Autodesk Inventor part; units mm, degrees
ref_plane "YZ Plane" through (0, 0, 0) normal (1, 0, 0) x (0, 1, 0)
ref_plane "XZ Plane" through (0, 0, 0) normal (0, 1, 0) x (-1, 0, 0)
ref_plane "XY Plane" through (0, 0, 0) normal (0, 0, 1) x (1, 0, 0)
sketch "Sketch1" plane through (0, 0, 0) normal (0, 1, 0) x (-1, 0, 0)
  point P0 (0, 0)
sketch "Sketch2" plane through (0, 0, 0) normal (0, 1, 0) x (-1, 0, 0)
  line L0 (0, 0) -> (-30, 0)
  line L1 (-30, 0) -> (-30, -30)
  line L2 (-30, -30) -> (0, -30)
  line L3 (0, -30) -> (0, 0)
  line L4 (0, -30) -> (-30, 0) construction
  line L5 (0, 0) -> (-30, -30) construction
  line L6 (-15, -15) -> (0, -15) construction
  line L7 (-15, -15) -> (-30, -15) construction
  line L8 (-15, -15) -> (-15, -30) construction
  line L9 (-15, -15) -> (-15, 0) construction
  line L10 (-15, -15) -> (-9.25, -15) construction
  line L11 (-15, -17.4158) -> (-15, -15) construction
  line L12 (-15, -15) -> (-15, -20.75) construction
  line L13 (-15, -15) -> (-15, -9.25) construction
  line L14 (-15, -15) -> (-9.25, -15) construction
  line L15 (-15, -15) -> (-20.75, -15) construction
  line L16 (-15, -20.75) -> (-9.25, -15) construction
  line L17 (-9.25, -15) -> (-9.25, -20.75) construction
  line L18 (-9.25, -20.75) -> (-15, -20.75) construction
  line L19 (-15, -20.75) -> (-20.75, -20.75) construction
  line L20 (-20.75, -20.75) -> (-20.75, -15) construction
  line L21 (-9.25, -15) -> (-9.25, -9.25) construction
  line L22 (-15, -9.25) -> (-9.25, -9.25) construction
  line L23 (-15, -9.25) -> (-20.75, -9.25) construction
  line L24 (-20.75, -9.25) -> (-20.75, -15) construction
  line L25 (-15, -9.25) -> (-11, -9.25) construction
  line L26 (-15, -9.25) -> (-19, -9.25) construction
  line L27 (-11, -9.25) -> (-19, -9.25)
  line L28 (-11, -9.25) -> (-11, -3.25)
  line L29 (-11, -3.25) -> (-19, -3.25)
  line L30 (-19, -3.25) -> (-19, -9.25)
  line L31 (-11, -20.75) -> (-19, -20.75)
  line L32 (-19, -20.75) -> (-19, -26.75)
  line L33 (-19, -26.75) -> (-11, -26.75)
  line L34 (-11, -26.75) -> (-11, -20.75)
  line L35 (-9.25, -9.25) -> (-9.25, -10.75)
  line L36 (-9.25, -20.75) -> (-9.25, -18.75)
  line L37 (-9.25, -18.75) -> (-9.25, -19.25)
  line L38 (-9.25, -18.75) -> (-9.25, -10.75)
  line L39 (-9.25, -10.75) -> (-3.25, -10.75)
  line L40 (-3.25, -10.75) -> (-3.25, -18.75)
  line L41 (-3.25, -18.75) -> (-9.25, -18.75)
  line L42 (-9.25, -19.25) -> (-20.75, -19.25) construction
  line L43 (-20.75, -19.25) -> (-20.75, -11.25)
  line L44 (-20.75, -11.25) -> (-26.75, -11.25)
  line L45 (-26.75, -11.25) -> (-26.75, -19.25)
  line L46 (-26.75, -19.25) -> (-20.75, -19.25)
  line L47 (-9.25, -18.75) -> (-11.75, -18.75) construction
  line L48 (-11.75, -18.75) -> (-11.75, -10.75) construction
  line L49 (-11.75, -10.75) -> (-9.25, -10.75) construction
  line L50 (-20.75, -19.25) -> (-18.25, -19.25) construction
  line L51 (-18.25, -19.25) -> (-18.25, -11.25) construction
  line L52 (-18.25, -11.25) -> (-20.75, -11.25) construction
  line L53 (-9.25, -10.75) -> (-9.25, -11.75) construction
  line L54 (-9.25, -11.75) -> (-11.75, -11.75) construction
  line L55 (-20.75, -11.25) -> (-20.75, -11.75) construction
  line L56 (-20.75, -11.75) -> (-18.25, -11.75) construction
  line L57 (-11.75, -18.75) -> (-20.75, -18.75) construction
  line L58 (-18.25, -18.75) -> (-18.25, -11.75) construction
  line L59 (-15, -18.75) -> (-14.25, -18.75) construction
  line L60 (-15, -18.75) -> (-15.75, -18.75) construction
  line L61 (-11.75, -18.75) -> (-11.75, -11.75)
  line L62 (-11.75, -18.75) -> (-14.25, -18.75)
  line L63 (-11.75, -11.75) -> (-14.25, -11.75)
  line L64 (-15.75, -18.75) -> (-18.25, -18.75)
  line L65 (-18.25, -18.75) -> (-18.25, -11.75)
  line L66 (-18.25, -11.75) -> (-15.75, -11.75)
  line L67 (-14.25, -11.75) -> (-15.75, -11.75)
  line L68 (-14.25, -18.75) -> (-15.75, -18.75)
  dimension "d0" = 30
  dimension "d1" = 30
  dimension "d3" = 5.75
  dimension "d4" = 5.75
  dimension "d5" = 5.75
  dimension "d6" = 5.75
  dimension "d7" = 4
  dimension "d8" = 4
  dimension "d9" = 6
  dimension "d10" = 6
  dimension "d11" = 8
  dimension "d12" = 1.5
  dimension "d13" = 2
  dimension "d14" = 0.5
  dimension "d15" = 6
  dimension "d16" = 8
  dimension "d17" = 6
  dimension "d18" = 2.5
  dimension "d19" = 2.5
  dimension "d20" = 1
  dimension "d21" = 0.75
  dimension "d22" = 0.75
extrude "Extrusion1" add sketch "Sketch2" against normal blind 5 contours L3 L2 L1 L0 | L62 L68 L64 L65 L66 L67 L63 L61
extrude "Extrusion5" cut sketch "Sketch2" against normal blind 4 contours L62 L68 L64 L65 L66 L67 L63 L61
properties part number "switch_test_v1_3DPrint"
Read the model definition and answer for the solid it produces. Units are mm, in the model's axes. A direction names the side the tool comes from. Give positions to 0.01 mm unless a question says otherwise; leave off trailing zeros. Write each loop counter-clockwise with the first axis right and the second up, starting at its lowest first coordinate (ties: lowest second). Pieces come first, ordered by that corner, then holes. Notation, with made-up numbers: (-38.75, 9.25) - (-33.75, 9.25) arc R10 ccw to (-33.75, 13.25) - close; hole circle Ø4 at (33.5, -12.75). An arc over 180 degrees is marked (long way). Answer in a Markdown table with one row per item. Add a question column.
Item 1: Determine the mould class of faces 1 (the face through (15, -2, 0)), 2 (the face through (30, -2, -15)), 3 (the face through (6, -2, -10.75)) for opening direction X: pulls with the +X half, pulls with the -X half, needs draft (parallel to the pull), parting line crosses it, or undercut.
Item 2: A tool of negligible diameter and unlimited length cuts with its end or side. For faces 4 (the face through (11, -2, -24)), 5 (the face through (15, -5, -15)), 6 (the face through (15, -2, -11.75)), from which of +Z, -Z, +X, -X, +Y, -Y can it reach the whole face along a straight path? Write none if from no direction.
Item 3: Section C-C, the plane x = 24.25 is taken. Write down the section's boundary in (y, z), and give its area (3 significant figures).
Item 4: Section B-B, the plane z = -7 is taken. Write down the section's boundary in (x, y).
Item 5: Section A-A, the plane y = -1.15 is taken. Write down the section's boundary in (x, z).
Item 6: Section D-D, the plane z = -14.75 is taken. Write down the section's boundary in (x, y), and give its area (3 significant figures).
Item 7: Find the intervals of material crossed by L1, parallel to X at y = -1.3, z = -13; L2, parallel to Z at x = 18.75, y = -3.8; L3, parallel to X at y = -2.9, z = -26.25, in increasing order.
Recorded:
| question | item | result |
|---|---|---|
| 1 | face 1 | needs draft |
| 1 | face 2 | pulls with the +X half |
| 1 | face 3 | undercut |
| 2 | face 4 | +Y, -Y |
| 2 | face 5 | +Z, -Z, +X, -X, -Y |
| 2 | face 6 | +Y |
| 3 | outline | (-5, -30) - (0, -30) - (0, -19.25) - (-5, -19.25) - close; (-5, -11.25) - (0, -11.25) - (0, 0) - (-5, 0) - close |
| 3 | area | 110 mm2 |
| 4 | outline | (0, -5) - (11, -5) - (11, 0) - (0, 0) - close; (19, -5) - (30, -5) - (30, 0) - (19, 0) - close |
| 5 | outline | (0, -30) - (30, -30) - (30, 0) - (0, 0) - close; hole (3.25, -18.75) - (9.25, -18.75) - (9.25, -10.75) - (3.25, -10.75) - close; hole (11, -26.75) - (19, -26.75) - (19, -20.75) - (11, -20.75) - close; hole (11, -9.25) - (19, -9.25) - (19, -3.25) - (11, -3.25) - close; hole (11.75, -18.75) - (18.25, -18.75) - (18.25, -11.75) - (11.75, -11.75) - close; hole (20.75, -19.25) - (26.75, -19.25) - (26.75, -11.25) - (20.75, -11.25) - close |
| 6 | outline | (0, -5) - (3.25, -5) - (3.25, 0) - (0, 0) - close; (9.25, -5) - (20.75, -5) - (20.75, 0) - (18.25, 0) - (18.25, -4) - (11.75, -4) - (11.75, 0) - (9.25, 0) - close; (26.75, -5) - (30, -5) - (30, 0) - (26.75, 0) - close |
| 6 | area | 64.0 mm2 |
| 7 | L1 | x = 0 to 3.25, 9.25 to 11.75, 18.25 to 20.75, 26.75 to 30 |
| 7 | L2 | z = -30 to -26.75, -20.75 to -9.25, -3.25 to 0 |
| 7 | L3 | x = 0 to 11, 19 to 30 |
